Geometry: final body of the model. Coordinates: model frame, mm. Round coordinates to 2 decimals unless told otherwise and drop trailing zeros. Loops run counter-clockwise (first coordinate to the right, second up) from the corner with the lowest first, then second, coordinate; pieces in that order, holes last. Notation, with made-up numbers: (64, 21.25) - (113, 21.25) arc R19 ccw to (113, 40.25) - close; hole circle Ø7 at (-21, 83). An arc over 180 degrees is marked (long way). Return JSON: item names as keys, results as strings. Group by question number.
1. Draft query along X for faces 1 (the face through (2082.8, -187, -94)), 2 (the face through (1027, 0, -7)), 3 (the face through (12.7, -142, -140)). Return one class per face: +X half, -X half, draft (parallel to the pull), parting line (faces both ways), or undercut.
2. First-contact query: pin 1 Ø4 at (x, y) = (1677.5, -200.5) entering from -Z; pin 2 Ø9.5 at (x, z) = (848.5, -19.5) entering from -Y; pin 3 Ø4 at (x, y) = (1195.5, -4.5) entering from -Z. Flat tips, straight axial feed; report the tip coordinate or a pass-through.
3. Section A-A on y = -185. Return loops of the section in (x, z), and give its area (3 significant figures).
4. Section C-C on x = 1416.5. Return loops of the section in (y, z).
5. Section B-B on z = -167. Return loops of the section in (x, y).
6. Material intervals for probe 1 along X at (y, z) = (-140, -140.5); probe 2 along Z at (x, y) = (1175, -108.5), sorted ascending.
from build123d import *

# Parameters (mm, degrees)
F0_W     = 2082.8
F0_H     = 304.8
F1_DEPTH = 19.05
F2_W     = 12.7
F2_H     = 31.75
F3_DEPTH = 2082.8
F5_DEPTH = 12.7
F7_DEPTH = 12.7


with BuildPart() as f1:
    # F0 (on Top) → F1 (new body)
    with BuildSketch(Plane.XY):
        with Locations((1041.4, -152.4)):
            Rectangle(F0_W, F0_H)
    extrude(amount=F1_DEPTH)

    # F2 (on Right) → F3 (join, through all)
    with BuildSketch(Plane.YZ):
        with Locations((-6.35, -15.875)):
            Rectangle(F2_W, F2_H)
    extrude(amount=F3_DEPTH)

    # F4 (on Right) → F5 (join)
    with BuildSketch(Plane.YZ):
        Polygon((-277.859232, 0), (-304.8, 0), (0, -304.8), (0, -277.859232), align=None)
    extrude(amount=F5_DEPTH)

    # F6 (on face) → F7 (join)
    with BuildSketch(Plane.YZ.offset(2082.8)):
        Polygon((0, -304.8), (0, -277.859232), (-277.859232, 0), (-304.8, 0), align=None)
    extrude(amount=-F7_DEPTH)


solid = f1.part
Taken from the geometry:
{
 "1": {"face 1": "+X half", "face 2": "draft", "face 3": "undercut"},
 "2": {"pin 1": "z = 0", "pin 2": "y = -12.7", "pin 3": "z = -31.75"},
 "3": {"outline": "(0, -119.8) - (12.7, -119.8) - (12.7, -92.86) - (0, -92.86) - close; (0, 0) - (2082.8, 0) - (2082.8, 19.05) - (0, 19.05) - close; (2070.1, -119.8) - (2082.8, -119.8) - (2082.8, -92.86) - (2070.1, -92.86) - close", "area": "40,400 mm2"},
 "4": {"outline": "(-304.8, 0) - (-12.7, 0) - (-12.7, -31.75) - (0, -31.75) - (0, 19.05) - (-304.8, 19.05) - close"},
 "5": {"outline": "(0, -137.8) - (12.7, -137.8) - (12.7, -110.86) - (0, -110.86) - close; (2070.1, -137.8) - (2082.8, -137.8) - (2082.8, -110.86) - (2070.1, -110.86) - close"},
 "6": {"probe 1": "0 to 12.7, 2070.1 to 2082.8", "probe 2": "0 to 19.05"}
}
